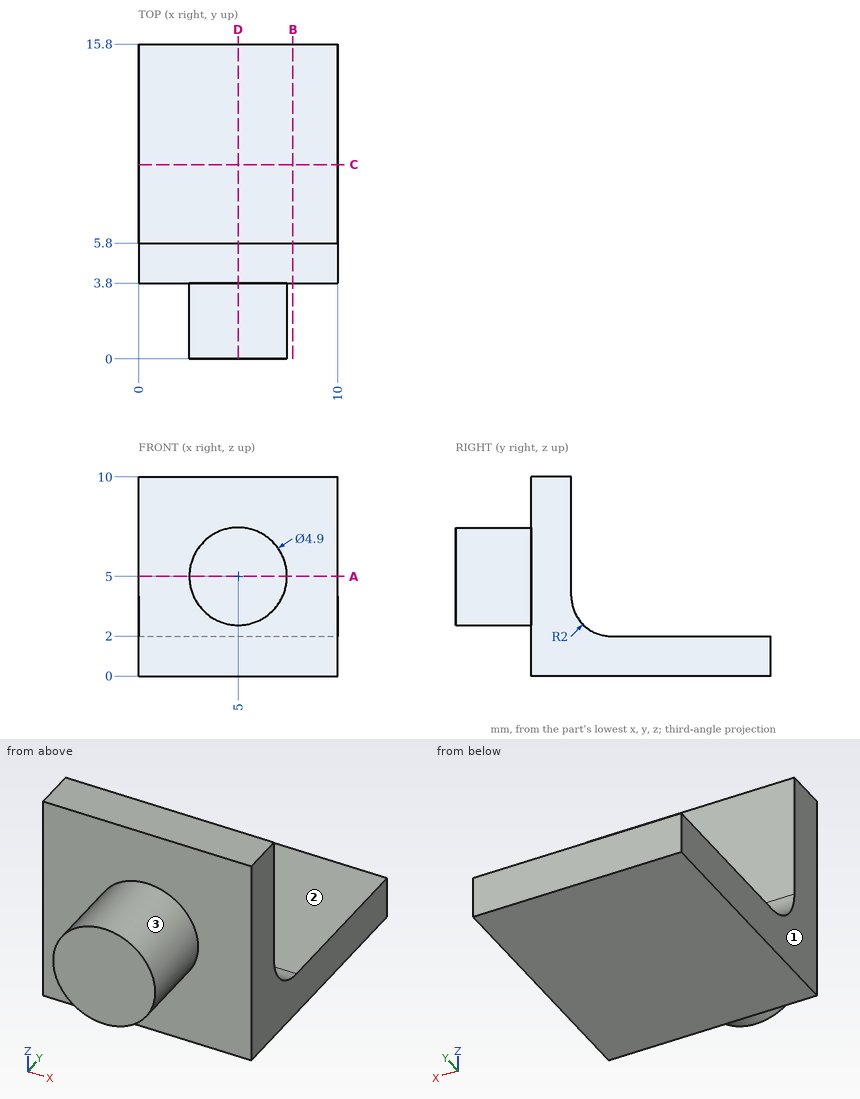
Print and shaded views of the part. All mm, measured from the part's lowest x, y and z. A direction names the side the tool comes from. Give positions to 0.01 mm unless a question says otherwise; leave off trailing zeros. Loops run counter-clockwise (first coordinate to the right, second up) from the corner with the lowest first, then second, coordinate; pieces in that order, holes last.
1) Saw through at D-D (x = 5). Write the cut outline in (y, z).
2) Saw through at B-B (x = 7.75). Write the cut outline in (y, z), plus the area to 3 significant figures.
3) Wall check: line 1 (Z direction, x = 2.75, y = 12.25); line 2 (Y direction, x = 3.5, z = 7.25); line 3 (Y direction, x = 4, z = 4.5). Give the ranges that are in metal, low to high.
4) Saw through at C-C (y = 9.75). Write the cut outline in (x, z), plus the area to 3 significant figures.
5) Flat gauge pins, fed straight in: pin 1 Ø5 at (x, y) = (7.5, 11) entering from +Z; pin 2 Ø2 at (x, y) = (2, 3) entering from -Z; pin 3 Ø5 at (x, z) = (5, 7) entering from +Y. Where does each tip first touch, or does it go through?
6) Tool access for the marked faces 1, 2 and 3: list every direction of +Z, -Z, +X, -X, +Y, -Y with a clear straight run to the whole face (end or side of a thin tool).
7) Saw through at A-A (z = 5). Write the cut outline in (x, y).
Answer block:
1. outline: (0, 2.55) - (3.8, 2.55) - (3.8, 0) - (15.8, 0) - (15.8, 2) - (7.8, 2) arc R2 cw to (5.8, 4) - (5.8, 10) - (3.8, 10) - (3.8, 7.45) - (0, 7.45) - close
2. outline: (3.8, 0) - (15.8, 0) - (15.8, 2) - (7.8, 2) arc R2 cw to (5.8, 4) - (5.8, 10) - (3.8, 10) - close
2. area: 40.9 mm2
3. line 1: z = 0 to 2
3. line 2: y = 3.8 to 5.8
3. line 3: y = 0 to 5.8
4. outline: (0, 0) - (10, 0) - (10, 2) - (0, 2) - close
4. area: 20.0 mm2
5. pin 1: stops at z = 2
5. pin 2: stops at z = 0
5. pin 3: stops at y = 5.8
6. face 1: +Z, -Z, -X, +Y, -Y
6. face 2: +Z, +X, -X, +Y
6. face 3: -Y
7. outline: (0, 3.8) - (2.55, 3.8) - (2.55, 0) - (7.45, 0) - (7.45, 3.8) - (10, 3.8) - (10, 5.8) - (0, 5.8) - close
